Part model, mm, in its own coordinate system. Face numbers are marked on the shaded views. A direction names the side the tool comes from. Give positions to 0.01 mm unless a question says otherwise; leave off trailing zeros. Write each loop counter-clockwise with the first axis right and the second up, starting at its lowest first coordinate (ties: lowest second). Pieces come first, ordered by that corner, then holes. Notation, with made-up numbers: (14.25, -38) - (42.25, -38) arc R14 ccw to (42.25, -30) - close; hole circle Ø3 at (35.5, 23.25). An arc over 180 degrees is marked (long way). Answer in a Markdown table with one row per item. Add a question column.
1. Band-saw the part on C-C on x = 8.5. Write the cut outline in (y, z).
2. Drop flat-ended pins along their axis: pin 1 Ø4.5 at (y, z) = (6.5, -19) entering from +X; pin 2 Ø1 at (y, z) = (9, -9.5) entering from +X; pin 3 Ø3 at (y, z) = (4, -16.5) entering from -X. Give the stop position or say it passes through.
3. Band-saw the part on A-A on z = 0. Write the cut outline in (x, y).
4. Which spindle directions (+Z, -Z, +X, -X, +Y, -Y) get a long thin tool onto all of the face, cutting with end or side? Do the marked faces 1, 2 and 3. Say none if no direction does.
5. Band-saw the part on B-B on y = 5. Write the cut outline in (x, z).
6. Band-saw the part on D-D on x = -10. Write the cut outline in (y, z), plus the area to 3 significant figures.
7. Probe line 1 along X through (y, z) = (3.25, 0); line 2 along X through (y, z) = (7.5, 9.5); line 3 along Z through (x, y) = (10, 2.5). List the from-to ranges inside material, lowest first.
8. Pull direction Y, two halves, no side cores. Call the marked faces 4, 5, 6 and 7: released by +Y, released by -Y, zero draft, split by the parting line, or undercut.
```python
from build123d import *

# Parameters (mm, degrees)
SALIENTE_EXTRUIR1_DEPTH = 10
REDONDEO1_R             = 1
REDONDEO2_R             = 2
CROQUIS2_R              = 3
CORTAR_EXTRUIR1_DEPTH   = 26.75


with BuildPart() as part:
    # Croquis1 → Saliente-Extruir1 (new body)
    with BuildSketch(Plane(origin=(0, 0, 0), x_dir=(1, 0, 0), z_dir=(0, 1, 0))):
        with BuildLine():
            Line((-9, 14.126659195), (-9, 25.619429464))
            Line((-9, 25.619429464), (-4, 25.619429464))
            Line((-4, 25.619429464), (-4, 14.974979132))
            ThreePointArc((-4, 14.974979132), (0, -15.5), (4, 14.974979132))
            Line((4, 14.974979132), (4, 25.619429464))
            Line((4, 25.619429464), (9, 25.619429464))
            Line((9, 25.619429464), (9, 14.126659195))
            ThreePointArc((9, 14.126659195), (0, -16.75), (-9, 14.126659195))
        make_face()
    extrude(amount=SALIENTE_EXTRUIR1_DEPTH)

    # Redondeo1
    redondeo1_edges = [part.edges().sort_by_distance(p)[0] for p in [
        (-4, 5, -14.974979132),
        (4, 5, -14.974979132),
    ]]
    fillet(redondeo1_edges, radius=REDONDEO1_R)

    # Redondeo2
    redondeo2_edges = [part.edges().sort_by_distance(p)[0] for p in [
        (-9, 5, -25.619429464),
        (-4, 5, -25.619429464),
        (4, 5, -25.619429464),
        (9, 5, -25.619429464),
    ]]
    fillet(redondeo2_edges, radius=REDONDEO2_R)

    # Croquis2 → Cortar-Extruir1 (cut, through all)
    with BuildSketch(Plane(origin=(9, 0, 0), x_dir=(0, 0, -1), z_dir=(1, 0, 0))):
        with Locations((18.873044329, 5)):
            Circle(CROQUIS2_R)
    extrude(amount=-CORTAR_EXTRUIR1_DEPTH, mode=Mode.SUBTRACT)


solid = part.part
```
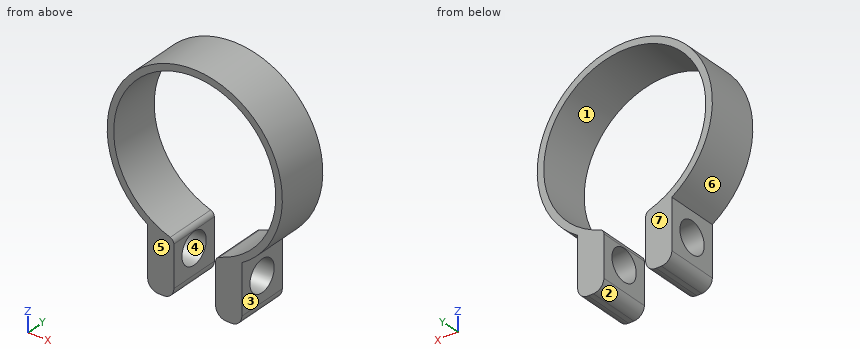
Values:
| question | item | result |
|---|---|---|
| 1 | outline | (0, -24.94) - (10, -24.94) - (10, -12.96) - (0, -12.96) - close; (0, 12.96) - (10, 12.96) - (10, 14.43) - (0, 14.43) - close; hole circle Ø6 at (5, -18.87) |
| 2 | pin 1 | stops at x = 9 |
| 2 | pin 2 | stops at x = 14.13 |
| 2 | pin 3 | stops at x = -9 |
| 3 | outline | (-16.75, 0) - (-15.5, 0) - (-15.5, 10) - (-16.75, 10) - close; (15.5, 0) - (16.75, 0) - (16.75, 10) - (15.5, 10) - close |
| 4 | face 1 | +Y, -Y |
| 4 | face 2 | -Z, +Y, -Y |
| 4 | face 3 | -Z, +X, +Y, -Y |
| 5 | outline | (-9, -23.62) arc R2 ccw to (-7, -25.62) - (-6, -25.62) arc R2 ccw to (-4, -23.62) - (-4, -21.87) - (-9, -21.87) - close; (-9, -15.87) - (-4, -15.87) - (-4, -15.72) arc R1 ccw to (-4.7, -14.77) arc R15.5 cw (long way) to (4.7, -14.77) arc R1 ccw to (4, -15.72) - (4, -15.87) - (9, -15.87) - (9, -14.13) arc R16.75 ccw (long way) to (-9, -14.13) - close; (4, -23.62) arc R2 ccw to (6, -25.62) - (7, -25.62) arc R2 ccw to (9, -23.62) - (9, -21.87) - (4, -21.87) - close |
| 6 | outline | (0, -13.44) - (10, -13.44) - (10, -11.84) - (0, -11.84) - close; (0, 11.84) - (10, 11.84) - (10, 13.44) - (0, 13.44) - close |
| 6 | area | 31.9 mm² |
| 7 | line 1 | x = -16.75 to -15.5, 15.5 to 16.75 |
| 7 | line 2 | x = -13.8 to -12.25, 12.25 to 13.8 |
| 7 | line 3 | z = -13.44 to -11.84, 11.84 to 13.44 |
| 8 | face 4 | undercut |
| 8 | face 5 | released by -Y |
| 8 | face 6 | zero draft |
| 8 | face 7 | released by +Y |
